```python
from build123d import *

# Parameters (mm, degrees)
SKETCH1_R           = 10
SKETCH1_R_2         = 1.5
BOSS_EXTRUDE1_DEPTH = 2.5
SKETCH2_R           = 4.5
BOSS_EXTRUDE2_DEPTH = 2
SKETCH3_R           = 2.6
CUT_EXTRUDE1_DEPTH  = 3.5
CHAMFER1_SIZE       = 0.2
FILLET1_R           = 0.2


with BuildPart() as part:
    # Sketch1 → Boss-Extrude1 (new body)
    with BuildSketch(Plane.XY):
        Circle(SKETCH1_R)
        with Locations((0, 7)):
            Circle(SKETCH1_R_2, mode=Mode.SUBTRACT)
        with Locations((7, 0)):
            Circle(SKETCH1_R_2, mode=Mode.SUBTRACT)
        with Locations((0, -7)):
            Circle(SKETCH1_R_2, mode=Mode.SUBTRACT)
        with Locations((-7, 0)):
            Circle(SKETCH1_R_2, mode=Mode.SUBTRACT)
        Circle(SKETCH1_R_2, mode=Mode.SUBTRACT)
    extrude(amount=BOSS_EXTRUDE1_DEPTH)

    # Sketch2 → Boss-Extrude2 (add)
    with BuildSketch(Plane.XY.offset(2.5)):
        Circle(SKETCH2_R)
    extrude(amount=BOSS_EXTRUDE2_DEPTH)

    # Sketch3 → Cut-Extrude1 (cut)
    with BuildSketch(Plane.XY.offset(4.5)):
        Circle(SKETCH3_R)
    extrude(amount=-CUT_EXTRUDE1_DEPTH, mode=Mode.SUBTRACT)

    # Chamfer1
    chamfer1_edges = [part.edges().sort_by_distance(p)[0] for p in [
        (-10, 0, 0),
        (-4.5, 0, 4.5),
        (-10, 0, 2.5),
    ]]
    chamfer(chamfer1_edges, length=CHAMFER1_SIZE)

    # Fillet1
    fillet1_edges = [part.edges().sort_by_distance(p)[0] for p in [
        (-4.5, 0, 2.5),
        (-2.6, 0, 1),
    ]]
    fillet(fillet1_edges, radius=FILLET1_R)


solid = part.part
```
Read the model definition and answer for the solid it produces. Units are mm, in the model's axes. A direction names the side the tool comes from. Give positions to 0.01 mm unless a question says otherwise; leave off trailing zeros. Order: outer loops, then holes, each group sorted by start corner. A loop starts at its lowest first (then second) coordinate and runs counter-clockwise, first axis right, second up.
(1) Straight lines are drawn through the part: L1, parallel to Y at x = 0, z = 1.35; L2, parallel to Y at x = 0, z = 0.7; L3, parallel to Z at x = -8, y = 2. For each, find the intervals that lie inside material, in ascending order.
(2) Find section A-A (y = 0). Give the number of separate pieces and of enclosed holes in the cut face, plus the area to 3 significant figures.
(3) Find section D-D (z = 4). Give the vertices of the cut face in (x, y).
(4) For faces 4 (the cylindrical face through (-8.5, 0.07, 1.23)), 5 (the flat face through (2, 4.5, 2.5)), determine the directions among +Z, -Z, +X, -X, +Y, -Y from which every point of the face is accessible in a straight line to the end or side of a thin tool.
(5) Given pin 1 (1 mm diameter, centred on x = 1.5, z = 1.5, fed in from +Y); pin 2 (2 mm diameter, centred on y = 5.5, z = 1.5, fed in from -X); pin 3 (1 mm diameter, centred on x = -6.5, z = 2.5, fed in from -Y), each flat-ended and moving along its own axis, determine where each tip first touches the part or whether it passes through.
(6) For a pull along X with two mould halves and no side action, classify faces 1 (the flat face through (0, -2, 1)), 2 (the cylindrical face through (-0.59, 4.46, 3.49)), 3 (the flat face through (2, 0, 0)) as released by +X, released by -X, zero draft, split by the parting line, or undercut.
(7) Find section B-B (z = 1.95). Give the vertices of the cut face in (x, y), plus the area to 3 significant figures.
Result sheet:
1. L1: y = -10 to -8.5, -5.5 to -2.6, 2.6 to 5.5, 8.5 to 10
1. L2: y = -10 to -8.5, -5.5 to -1.5, 1.5 to 5.5, 8.5 to 10
1. L3: z = 0 to 2.5
2. separate pieces: 4
2. enclosed holes: 0
2. area: 31.7 mm2
3. outline: circle Ø9 at (0, 0); hole circle Ø5.2 at (0, 0)
4. face 4: +Z, -Z
4. face 5: +Z
5. pin 1: stops at y = 9.95
5. pin 2: stops at x = -8.93
5. pin 3: stops at y = -7.97
6. face 1: undercut
6. face 2: split by the parting line
6. face 3: zero draft
7. outline: circle Ø20 at (0, 0); hole circle Ø3 at (-7, 0); hole circle Ø5.2 at (0, 0); hole circle Ø3 at (0, -7); hole circle Ø3 at (0, 7); hole circle Ø3 at (7, 0)
7. area: 265 mm2
